from build123d import *

# Parameters (mm, degrees)
ESQUISSE1_W                  = 95
ESQUISSE1_H                  = 65
BOSS_EXTRU_1_DEPTH           = 83
ENL_V_MAT_EXTRU_3_DEPTH      = 30.5
ENL_V_MAT_EXTRU_3_DEPTH_BACK = 30.5
ESQUISSE4_W                  = 91
ESQUISSE4_H                  = 79
ESQUISSE2_R                  = 1.1
ESQUISSE2_R_2                = 3.25
ESQUISSE2_W                  = 20
ESQUISSE2_H                  = 12.18
ESQUISSE2_W_2                = 3
ESQUISSE2_H_2                = 10.1
ENL_V_MAT_EXTRU_1_DEPTH      = 10
ESQUISSE5_R                  = 3.05
ENL_V_MAT_EXTRU_4_DEPTH      = 10
ESQUISSE6_W                  = 13
ESQUISSE6_H                  = 13
ENL_V_MAT_EXTRU_6_DEPTH      = 10
R_P_TITION_LIN_AIRE1_COUNT   = 2
R_P_TITION_LIN_AIRE1_PITCH   = 20
ENL_V_MAT_EXTRU_7_REACH      = 132.27
ESQUISSE9_W                  = 3
ESQUISSE9_H                  = 65
BOSS_EXTRU_2_DEPTH           = 16
ESQUISSE11_R                 = 2
ENL_V_MAT_EXTRU_8_DEPTH      = 4
CHANFREIN5_SIZE              = 10
CHANFREIN6_SIZE              = 10
CHANFREIN7_SIZE              = 10
CHANFREIN8_SIZE              = 10


with BuildPart() as part:
    # Esquisse1 → Boss.-Extru.1 (new body)
    with BuildSketch(Plane.XY):
        Rectangle(ESQUISSE1_W, ESQUISSE1_H)
    extrude(amount=BOSS_EXTRU_1_DEPTH)

    # Esquisse4 → Enlèv. mat.-Extru.3 (cut, two sides: drawn at the far end of the back side and taken through both)
    with BuildSketch(Plane(origin=(0, 0, 0), x_dir=(1, 0, 0), z_dir=(0, 1, 0)).offset(-ENL_V_MAT_EXTRU_3_DEPTH_BACK)):
        with Locations((0, -41.5)):
            Rectangle(ESQUISSE4_W, ESQUISSE4_H)
    extrude(amount=ENL_V_MAT_EXTRU_3_DEPTH + ENL_V_MAT_EXTRU_3_DEPTH_BACK, mode=Mode.SUBTRACT)

    # Esquisse2 → Enlèv. mat.-Extru.1 (cut)
    with BuildSketch(Plane.XY.offset(83)):
        with Locations((-39.5, 0)):
            Circle(ESQUISSE2_R)
        with Locations((-39.5, -20.7)):
            Circle(ESQUISSE2_R)
        with Locations((-16.30439307, 0)):
            Circle(ESQUISSE2_R)
        with Locations((-16.30439307, -20.7)):
            Circle(ESQUISSE2_R)
        with Locations((3.01560693, 10)):
            Circle(ESQUISSE2_R_2)
        with Locations((3.01560693, -10)):
            Circle(ESQUISSE2_R_2)
        with Locations((-27.5, 18.41)):
            Rectangle(ESQUISSE2_W, ESQUISSE2_H)
        with Locations((-39, -10.1)):
            Rectangle(ESQUISSE2_W_2, ESQUISSE2_H_2)
    extrude(amount=-ENL_V_MAT_EXTRU_1_DEPTH, mode=Mode.SUBTRACT)

    # Esquisse5 → Enlèv. mat.-Extru.4 (cut)
    with BuildSketch(Plane(origin=(47.5, 0, 0), x_dir=(0, 0, -1), z_dir=(1, 0, 0))):
        with Locations((-68, -22)):
            Circle(ESQUISSE5_R)
        with Locations((-68, -10)):
            Circle(ESQUISSE5_R)
        with Locations((-53, -22)):
            Circle(ESQUISSE5_R)
        with Locations((-53, -10)):
            Circle(ESQUISSE5_R)
        with Locations((-38, -22)):
            Circle(ESQUISSE5_R)
        with Locations((-38, -10)):
            Circle(ESQUISSE5_R)
        with Locations((-68, 8)):
            Circle(ESQUISSE5_R)
        with Locations((-68, 20)):
            Circle(ESQUISSE5_R)
        with Locations((-53, 20)):
            Circle(ESQUISSE5_R)
        with Locations((-53, 8)):
            Circle(ESQUISSE5_R)
        with Locations((-38, 20)):
            Circle(ESQUISSE5_R)
        with Locations((-38, 8)):
            Circle(ESQUISSE5_R)
    extrude(amount=-ENL_V_MAT_EXTRU_4_DEPTH, mode=Mode.SUBTRACT)

    # Esquisse6 → Enlèv. mat.-Extru.6 (cut)
    with BuildSketch(Plane(origin=(47.5, 0, 0), x_dir=(0, 0, -1), z_dir=(1, 0, 0))):
        with Locations((-12, -10)):
            Rectangle(ESQUISSE6_W, ESQUISSE6_H)
    extrude(amount=-ENL_V_MAT_EXTRU_6_DEPTH, mode=Mode.SUBTRACT)

    # Esquisse8 → Dégagement M101 (revolve, cut)
    with BuildSketch(Plane(origin=(23.69560693, 10, 83), x_dir=(0, -1, 0), z_dir=(1, 0, 0))):
        Polygon((0, 0), (0, 21.474733405), (5.5, 18.17), (5.5, 0.025), (5.525, 0), align=None)
    d_gagement_m101 = revolve(axis=Axis((23.69560693, 10, 89.35), (0, 0, -1)), mode=Mode.SUBTRACT)

    # Répétition linéaire1: Dégagement M101 ×2
    with Locations(*[(0, -i * R_P_TITION_LIN_AIRE1_PITCH, 0) for i in range(1, R_P_TITION_LIN_AIRE1_COUNT)]):
        add(d_gagement_m101, mode=Mode.SUBTRACT)

    # Esquisse9 → Enlèv. mat.-Extru.7 (cut, up to next)
    with BuildSketch(Plane(origin=(47.5, 0, 0), x_dir=(0, 0, -1), z_dir=(1, 0, 0)), mode=Mode.PRIVATE) as enl_v_mat_extru_7_sk1:
        with Locations((-1.5, 0)):
            Rectangle(ESQUISSE9_W, ESQUISSE9_H)
    enl_v_mat_extru_7_tool1 = extrude(enl_v_mat_extru_7_sk1.sketch, amount=-ENL_V_MAT_EXTRU_7_REACH, mode=Mode.PRIVATE) & part.part
    add(enl_v_mat_extru_7_tool1.solids().sort_by_distance((47.5, 0, 1.5))[0], mode=Mode.SUBTRACT)

    # Esquisse10 → Boss.-Extru.2 (add)
    with BuildSketch(Plane(origin=(0, 0, 3), x_dir=(-1, 0, 0), z_dir=(0, 0, -1))):
        Polygon((-45.5, 16.5), (-31.5, 30.5), (-45.5, 30.5), align=None)
        Polygon((45.5, 16.5), (31.5, 30.5), (45.5, 30.5), align=None)
        Polygon((45.5, -16.5), (31.5, -30.5), (45.5, -30.5), align=None)
        Polygon((-45.5, -16.5), (-31.5, -30.5), (-45.5, -30.5), align=None)
    extrude(amount=-BOSS_EXTRU_2_DEPTH)

    # Esquisse11 → Enlèv. mat.-Extru.8 (cut)
    with BuildSketch(Plane(origin=(0, 0, 3), x_dir=(-1, 0, 0), z_dir=(0, 0, -1))):
        with Locations(Location((-41.5, 26.5, 0), (0, 0, 90))):
            Circle(ESQUISSE11_R)
        with Locations(Location((41.5, 26.5, 0), (0, 0, 270))):
            Circle(ESQUISSE11_R)
        with Locations(Location((-41.5, -26.5, 0), (0, 0, 270))):
            Circle(ESQUISSE11_R)
        with Locations(Location((41.5, -26.5, 0), (0, 0, 90))):
            Circle(ESQUISSE11_R)
    extrude(amount=-ENL_V_MAT_EXTRU_8_DEPTH, mode=Mode.SUBTRACT)

    # Chanfrein5
    # the kernel refuses this chamfer: 10 mm, written as the material it takes off along each edge
    with BuildSketch(Plane(origin=(63.684544799, -1.684544799, 19), x_dir=(-0.019442520806014222, -0.019442520806014142, -0.9996219169112968), z_dir=(-0.7071067811865474, 0.7071067811865478, 0))) as chanfrein5_piece_1_section:
        Polygon((CHANFREIN5_SIZE * 0.999621916911, -CHANFREIN5_SIZE * 0.0274958766106), (-CHANFREIN5_SIZE * 0.0274958766106, -CHANFREIN5_SIZE * 0.999621916911), (0, 0), align=None)
    chanfrein5_piece_1 = extrude(amount=71.232649633, mode=Mode.PRIVATE)
    chanfrein5_piece_1 = split(chanfrein5_piece_1, bisect_by=Plane(origin=(45.5, 25.258750221, 15.243624208), z_dir=(-1, 0, 0)), keep=Keep.TOP, mode=Mode.PRIVATE)
    chanfrein5_piece_1 = split(chanfrein5_piece_1, bisect_by=Plane(origin=(40.258750221, 30.5, 15.243624208), z_dir=(0, -1, 0)), keep=Keep.TOP, mode=Mode.PRIVATE)
    add(chanfrein5_piece_1, mode=Mode.SUBTRACT)

    # Chanfrein6
    # the kernel refuses this chamfer: 10 mm, written as the material it takes off along each edge
    with BuildSketch(Plane(origin=(-63.684544799, 1.684544799, 19), x_dir=(0.019442520806014323, 0.01944252080601439, -0.9996219169112968), z_dir=(0.7071067811865476, -0.7071067811865476, 0))) as chanfrein6_piece_1_section:
        Polygon((CHANFREIN6_SIZE * 0.999621916911, -CHANFREIN6_SIZE * 0.0274958766106), (-CHANFREIN6_SIZE * 0.0274958766106, -CHANFREIN6_SIZE * 0.999621916911), (0, 0), align=None)
    chanfrein6_piece_1 = extrude(amount=71.232649633, mode=Mode.PRIVATE)
    chanfrein6_piece_1 = split(chanfrein6_piece_1, bisect_by=Plane(origin=(-45.5, -25.258750221, 15.243624208), z_dir=(1, 0, 0)), keep=Keep.TOP, mode=Mode.PRIVATE)
    chanfrein6_piece_1 = split(chanfrein6_piece_1, bisect_by=Plane(origin=(-40.258750221, -30.5, 15.243624208), z_dir=(0, 1, 0)), keep=Keep.TOP, mode=Mode.PRIVATE)
    add(chanfrein6_piece_1, mode=Mode.SUBTRACT)

    # Chanfrein7
    # the kernel refuses this chamfer: 10 mm, written as the material it takes off along each edge
    with BuildSketch(Plane(origin=(63.684544799, 1.684544799, 19), x_dir=(0.7068394360706736, -0.7068394360706736, 0.02749587661058597), z_dir=(-0.7071067811865476, -0.7071067811865476, 0))) as chanfrein7_piece_1_section:
        Polygon((CHANFREIN7_SIZE * 0.999621916911, -CHANFREIN7_SIZE * 0.0274958766106), (-CHANFREIN7_SIZE * 0.0274958766106, -CHANFREIN7_SIZE * 0.999621916911), (0, 0), align=None)
    chanfrein7_piece_1 = extrude(amount=71.232649633, mode=Mode.PRIVATE)
    chanfrein7_piece_1 = split(chanfrein7_piece_1, bisect_by=Plane(origin=(40.831369683, -30.5, 18.750065142), z_dir=(0, 1, 0)), keep=Keep.TOP, mode=Mode.PRIVATE)
    chanfrein7_piece_1 = split(chanfrein7_piece_1, bisect_by=Plane(origin=(45.5, -25.831369683, 18.750065142), z_dir=(-1, 0, 0)), keep=Keep.TOP, mode=Mode.PRIVATE)
    add(chanfrein7_piece_1, mode=Mode.SUBTRACT)

    # Chanfrein8
    # the kernel refuses this chamfer: 10 mm, written as the material it takes off along each edge
    with BuildSketch(Plane(origin=(-63.684544799, -1.684544799, 19), x_dir=(0.019442520806014378, -0.019442520806014312, -0.9996219169112968), z_dir=(0.7071067811865476, 0.7071067811865476, 0))) as chanfrein8_piece_1_section:
        Polygon((CHANFREIN8_SIZE * 0.999621916911, CHANFREIN8_SIZE * 0.0274958766106), (-CHANFREIN8_SIZE * 0.0274958766106, CHANFREIN8_SIZE * 0.999621916911), (0, 0), align=None)
    chanfrein8_piece_1 = extrude(amount=71.232649633, mode=Mode.PRIVATE)
    chanfrein8_piece_1 = split(chanfrein8_piece_1, bisect_by=Plane(origin=(-45.5, 25.258750221, 15.243624208), z_dir=(1, 0, 0)), keep=Keep.TOP, mode=Mode.PRIVATE)
    chanfrein8_piece_1 = split(chanfrein8_piece_1, bisect_by=Plane(origin=(-40.258750221, 30.5, 15.243624208), z_dir=(0, -1, 0)), keep=Keep.TOP, mode=Mode.PRIVATE)
    add(chanfrein8_piece_1, mode=Mode.SUBTRACT)


solid = part.part
Could you check a few things on this model? Use its own coordinates, in mm. A direction names the side the tool comes from. Coordinates: 2 decimals unless noted, no trailing zeros. Loops run counter-clockwise (first coordinate to the right, second up) from the corner with the lowest first, then second, coordinate; pieces in that order, holes last. Notation, with made-up numbers: (-20, 77) -> (2, 77) arc R27 ccw to (2, 112) -> close; hole circle Ø1 at (7.5, -4.75). An arc over 180 degrees is marked (long way). Answer in a Markdown table with one row per item.
(1) Thinking about a two-plate mould opening in Y: for faces 6 (the face through (46.514, 20.134, 56.047)), 7 (the face through (-1, -32.5, 42)), 8 (the face through (0, -31, 3)), which applies, released by +Y, released by -Y, zero draft, split by the parting line, or undercut?
Results found:
| item | result |
|---|---|
| face 6 | undercut |
| face 7 | released by -Y |
| face 8 | zero draft |
(2) For faces 1 (the face through (46.514, -9.866, 71.047)), 2 (the face through (39, 23, 6)), 3 (the face through (-1, 32.5, 42)), 4 (the face through (2.59, 13.22, 82.01)), 5 (the face through (-1, -30.5, 41)), which set-ups out of +Z, -Z, +X, -X, +Y, -Y let a thin tool reach every point of the face, with its end or its side?
Results found:
| item | result |
|---|---|
| face 1 | +X |
| face 2 | -Z |
| face 3 | +Z, -Z, +X, -X, +Y |
| face 4 | +Z, -Z |
| face 5 | none |
(3) Will these pins go through, and if not, where does the flat tip stop? pin 1 Ø1.2 at (x, y) = (-42.5, -26.5) entering from -Z; pin 2 Ø10 at (x, y) = (-5.5, -15) entering from -Z; pin 3 Ø5 at (y, z) = (-10, 68) entering from +X.
Results found:
| item | result |
|---|---|
| pin 1 | stops at z = 7 |
| pin 2 | stops at z = 81 |
| pin 3 | stops at x = -45.5 |
(4) Imagine slicing it at A-A (x = -29). List the corners of the cut face in (y, z) for me.
Results found:
| item | result |
|---|---|
| outline | (-32.5, 3) -> (-30.5, 3) -> (-30.5, 81) -> (12.32, 81) -> (12.32, 83) -> (-32.5, 83) -> close; (24.5, 81) -> (30.5, 81) -> (30.5, 3) -> (32.5, 3) -> (32.5, 83) -> (24.5, 83) -> close |
(5) Imagine slicing it at C-C (z = 73). List the corners of the cut face in (x, y) for me.
Results found:
| item | result |
|---|---|
| outline | (-47.5, -32.5) -> (47.5, -32.5) -> (47.5, 32.5) -> (-47.5, 32.5) -> close; hole (-45.5, -30.5) -> (45.5, -30.5) -> (45.5, 30.5) -> (-45.5, 30.5) -> close |
(6) Imagine slicing it at B-B (z = 53). List the corners of the cut face in (x, y) for me.
Results found:
| item | result |
|---|---|
| outline | (-47.5, -32.5) -> (47.5, -32.5) -> (47.5, -25.05) -> (45.5, -25.05) -> (45.5, -30.5) -> (-45.5, -30.5) -> (-45.5, 30.5) -> (45.5, 30.5) -> (45.5, 23.05) -> (47.5, 23.05) -> (47.5, 32.5) -> (-47.5, 32.5) -> close; (45.5, -18.95) -> (47.5, -18.95) -> (47.5, -13.05) -> (45.5, -13.05) -> close; (45.5, -6.95) -> (47.5, -6.95) -> (47.5, 4.95) -> (45.5, 4.95) -> close; (45.5, 11.05) -> (47.5, 11.05) -> (47.5, 16.95) -> (45.5, 16.95) -> close |
(7) Imagine slicing it at D-D (x = -13.5). List the corners of the cut face in (y, z) for me, plus the area to 3 significant figures.
Results found:
| item | result |
|---|---|
| outline | (-32.5, 3) -> (-30.5, 3) -> (-30.5, 81) -> (30.5, 81) -> (30.5, 3) -> (32.5, 3) -> (32.5, 83) -> (-32.5, 83) -> close |
| area | 442 mm^2 |
(8) If I drill on probe 1 along Y at (x, z) = (46.1, 53); probe 2 along Y at (x, z) = (-33, 13); probe 3 along X at (y, z) = (15, 59.5), over which ranges is the centre line in solid material (lowest first)?
Results found:
| item | result |
|---|---|
| probe 1 | y = -32.5 to -25.05, -18.95 to -13.05, -6.95 to 4.95, 11.05 to 16.95, 23.05 to 32.5 |
| probe 2 | y = -32.5 to -30.5, 30.5 to 32.5 |
| probe 3 | x = -47.5 to -45.5, 45.5 to 47.5 |
